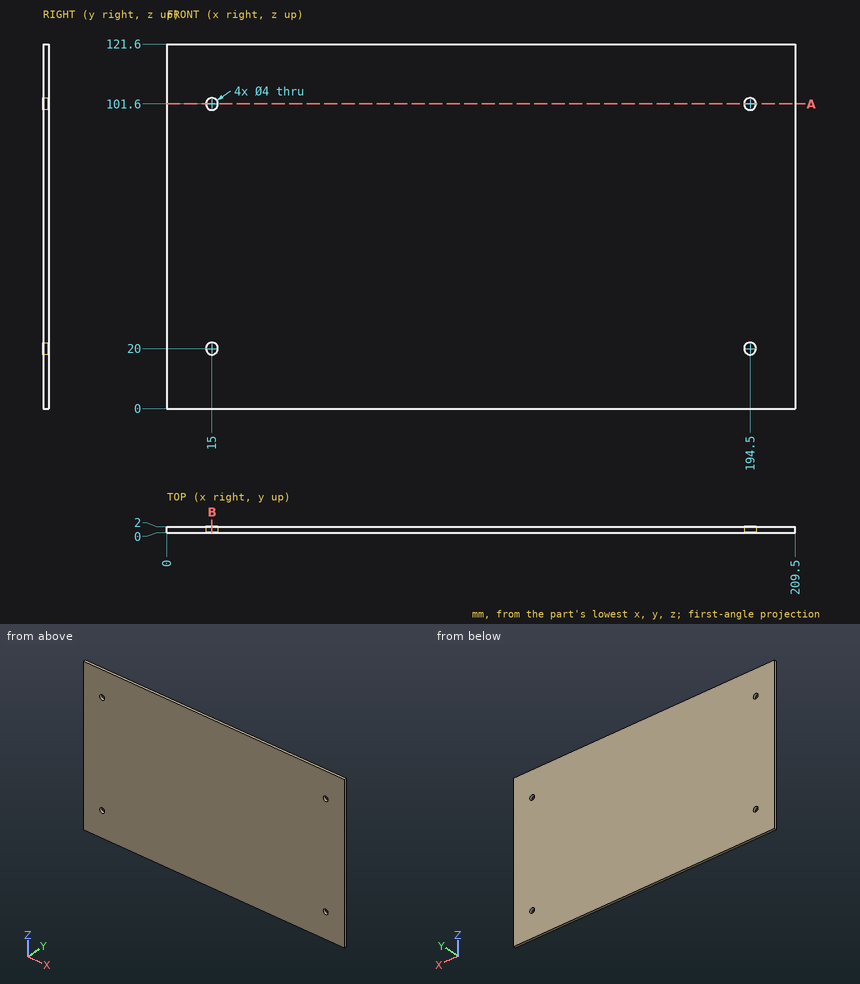
Drawing for the job (mm, zero at the part's lowest x, y, z). Round coordinates to 2 decimals unless told otherwise and drop trailing zeros. Order: outer loops, then holes, each group sorted by start corner. A loop starts at its lowest first (then second) coordinate and runs counter-clockwise, first axis right, second up. Notation, with made-up numbers: (71, 1.5) -> (79, 1.5) arc R10 ccw to (79, 7.5) -> close; hole circle Ø7 at (-16.5, -26.5). An arc over 180 degrees is marked (long way). Write item = value, one per line. Start each with the question number.
(1) Cut at A-A, the plane z = 101.6. List the corners of the cut face in (x, y), then the cut area to 3 significant figures.
(2) Cut at B-B, the plane x = 15. List the corners of the cut face in (y, z).
(3) Probe line 1 (X direction, y = 0.8, z = 20); line 2 (Z direction, x = 194.5, y = 0.5). List the from-to ranges inside material, lowest first. Write a range as [from, to].
Model answer:
q1.outline = (0, 0) -> (13, 0) -> (13, 2) -> (0, 2) -> close; (17, 0) -> (192.5, 0) -> (192.5, 2) -> (17, 2) -> close; (196.5, 0) -> (209.5, 0) -> (209.5, 2) -> (196.5, 2) -> close
q1.area = 403 mm2
q2.outline = (0, 0) -> (2, 0) -> (2, 18) -> (0, 18) -> close; (0, 22) -> (2, 22) -> (2, 99.6) -> (0, 99.6) -> close; (0, 103.6) -> (2, 103.6) -> (2, 121.6) -> (0, 121.6) -> close
q3.line_1 = [0, 13], [17, 192.5], [196.5, 209.5]
q3.line_2 = [0, 18], [22, 99.6], [103.6, 121.6]
